Check sheet for the drawn part. Datum: minimum x, y, z corner. Units: mm. A direction names the side the tool comes from. Coordinates: 2 decimals unless noted, no trailing zeros. Write each loop counter-clockwise with the first axis right and the second up, starting at its lowest first coordinate (ties: lowest second). Pieces come first, ordered by that corner, then holes. Notation, with made-up numbers: (-39, 58) - (-8, 58) arc R16 ccw to (-8, 87) - close; hole circle Ø5 at (-26, 79.5). An arc over 180 degrees is marked (long way). Use CSV: the item, a comma, the result in double quotes. Start each with the question number.
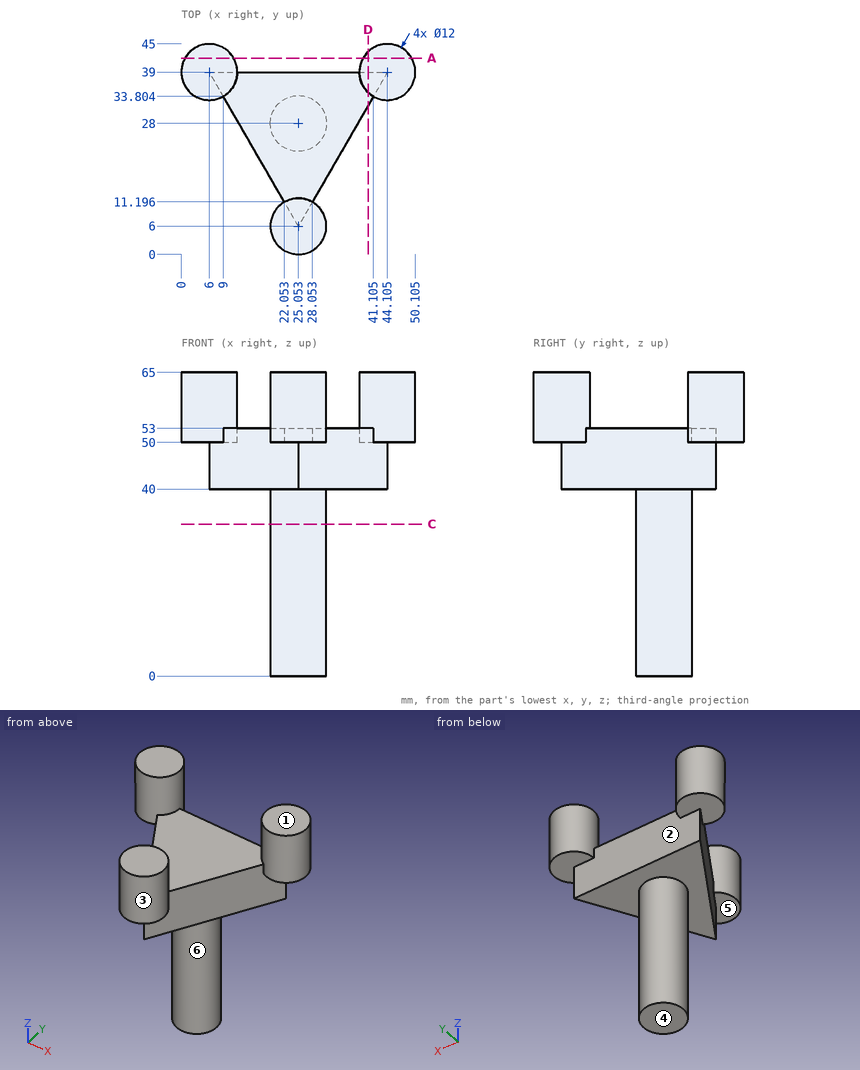
Q1. Cross-section at D-D (x = 40). Record the cut outline in (y, z) (1 decimal).
Q2. Scan lines: line 1 along Z through (x, y) = (22, 4.5); line 2 along Z through (x, y) = (30.5, 23); line 3 along Y through (x, z) = (33.5, 51) (1 decimal). Record each from-to range of solid material in increasing order. Write a range as from..to.
Q3. Release check for a two-part mould opening along X. For the marked faces 1, 2 and 3 record: released by +X, released by -X, zero draft, split by the parting line, or undercut.
Q4. Gauge pin test, flat ends, axial feed: pin 1 (12 mm diameter, centred on y = 13.5, z = 49.5, fed in from -X); pin 2 (4 mm diameter, centred on x = 43.5, y = 37, fed in from -Z); pin 3 (2 mm diameter, centred on x = 29, y = 37.5, fed in from +Z). Record the tip position at first contact, or that the pin passes through.
Q5. Cross-section at C-C (z = 32.5). Record the cut outline in (x, y).
Q6. Tool access check on the marked faces 4, 5 and 6. Record the directions out of +Z, -Z, +X, -X, +Y, -Y that give a thin tool (end or side, any length) a straight path to the whole face; none if there is none.
Q7. Cross-section at A-A (y = 42). Record the cut outline in (x, z).
Reply:
1,outline,"(31.9, 40) - (39, 40) - (39, 50) - (43.4, 50) - (43.4, 65) - (34.6, 65) - (34.6, 53) - (31.9, 53) - close"
2,line 1,"50..65"
2,line 2,"40..53"
2,line 3,"20.6..39"
3,face 1,"zero draft"
3,face 2,"undercut"
3,face 3,"split by the parting line"
4,pin 1,"x = 17.26"
4,pin 2,"z = 40"
4,pin 3,"z = 53"
5,outline,"circle Ø12 at (25.05, 28)"
6,face 4,"-Z, +X, -X, +Y, -Y"
6,face 5,"-Z, -Y"
6,face 6,"-Z"
7,outline,"(0.8, 50) - (11.2, 50) - (11.2, 65) - (0.8, 65) - close; (38.91, 50) - (49.3, 50) - (49.3, 65) - (38.91, 65) - close"
